For this review, take the finished solid that the model builds, in its own axes (mm). A direction names the side the tool comes from. Coordinates: 2 decimals unless noted, no trailing zeros. Write each loop counter-clockwise with the first axis right and the second up, starting at its lowest first coordinate (ties: lowest second). Pieces come first, ordered by that corner, then holes. Notation, with made-up numbers: (38, 84.5) -> (45, 84.5) arc R20 ccw to (45, 89.5) -> close; hole circle Ø5 at (-32, -8.75). An arc over 180 degrees is marked (long way). Put each result on its own line as item: value. Start each with the question number.
Item 1: For faces 5 (the flat face through (12, -3, 1)), 6 (the cylindrical face through (17.456, 0.011, 3.857)), list the 3-axis set-ups (+Z, -Z, +X, -X, +Y, -Y) from which the entire face can be reached by the end or side of a thin tool; tool diameter is ignored.
Item 2: Consider section A-A on x = 16.25. Give the boundary of the cut face in (y, z).
Item 3: Insertion check: P1, Ø1.8, axis at x = 15, z = 4, coming from the +Y side; P2, Ø2.5, axis at x = 15.5, z = 3.5, coming from the -Y side. Each pin has a flat end and moves straight along its axis. Give the tip position at first contact, or say it passes through.
Item 4: Consider section C-C on y = -0.25. Give the boundary of the cut face in (x, z).
Item 5: Consider section B-B on z = 1.6. Give the boundary of the cut face in (x, y), and give its area (3 significant figures).
Item 6: The part is to be moulded in two halves that separate along X. For faces 1 (the flat face through (15, 0.5, 4)), 2 (the flat face through (18.456, 0, 3)), 3 (the flat face through (12, 0, 0)), 4 (the flat face through (15, -0.5, 4)), say which applies: +X half, -X half, draft (parallel to the pull), parting line (faces both ways), or undercut.
Item 7: To check wall thickness, follow L1, parallel to Y at x = 15.75, z = 0.4; L2, parallel to X at y = 0.25, z = 4.15; L3, parallel to Y at x = 18, z = 2.45. State the ranges of each line that lie inside material, in increasing order.
```python
from build123d import *

# Parameters (mm, degrees)
F0_W     = 12
F0_H     = 6
F1_DEPTH = 5
F2_R     = 2.99999
F3_R     = 1.25
F4_DEPTH = 25
F6_DEPTH = 25


# Not quite as in the source:
# - a fillet or chamfer is up to 0.001 mm smaller than in the source, because OpenCascade refuses the exact size


with BuildPart() as f1:
    # F0 (on Top) → F1 (new body)
    with BuildSketch(Plane.XY):
        with Locations((12.4557307512, 0)):
            Rectangle(F0_W, F0_H)
    extrude(amount=F1_DEPTH)

    # F2 (radius 3 in the source; OpenCascade refuses exactly that, so slightly less here)
    f2_edges = [f1.edges().sort_by_distance(p)[0] for p in [
        (12.455731, -3, 5),
        (12.455731, 3, 5),
    ]]
    fillet(f2_edges, radius=F2_R)

    # F3 (on face) → F4 (cut)
    with BuildSketch(Plane.YZ.offset(18.4557307512)):
        with Locations((0, 1.6)):
            Circle(F3_R)
    extrude(amount=-F4_DEPTH, mode=Mode.SUBTRACT)

    # F5 (on face) → F6 (cut)
    with BuildSketch(Plane(origin=(0, 0, 0), x_dir=(1, 0, 0), z_dir=(0, 0, -1))):
        with BuildLine():
            Line((13.9557307512, -0.5), (16.9557307512, -0.5))
            ThreePointArc((16.9557307512, -0.5), (17.4557307512, 0), (16.9557307512, 0.5))
            Line((16.9557307512, 0.5), (13.9557307512, 0.5))
            ThreePointArc((13.9557307512, 0.5), (13.4557307512, 0), (13.9557307512, -0.5))
        make_face()
    extrude(amount=-F6_DEPTH, mode=Mode.SUBTRACT)


solid = f1.part
```
Return value:
1. face 5: +Z, -Z, +X, -X, -Y
1. face 6: +Z, -Z
2. outline: (-3, 0) -> (-0.5, 0) -> (-0.5, 0.45) arc R1.25 cw to (-0.5, 2.75) -> (-0.5, 4.96) arc R3 ccw to (-3, 2) -> close; (0.5, 0) -> (3, 0) -> (3, 2) arc R3 ccw to (0.5, 4.96) -> (0.5, 2.75) arc R1.25 cw to (0.5, 0.45) -> close
3. P1: y = 2.79
3. P2: y = -2.99
4. outline: (6.46, 0) -> (13.52, 0) -> (13.52, 0.38) -> (6.46, 0.38) -> close; (6.46, 2.82) -> (13.52, 2.82) -> (13.52, 4.99) -> (6.46, 4.99) -> close; (17.39, 0) -> (18.46, 0) -> (18.46, 0.38) -> (17.39, 0.38) -> close; (17.39, 2.82) -> (18.46, 2.82) -> (18.46, 4.99) -> (17.39, 4.99) -> close
5. outline: (6.46, -3) -> (18.46, -3) -> (18.46, -1.25) -> (6.46, -1.25) -> close; (6.46, 1.25) -> (18.46, 1.25) -> (18.46, 3) -> (6.46, 3) -> close
5. area: 42.0 mm^2
6. face 1: undercut
6. face 2: +X half
6. face 3: draft
6. face 4: undercut
7. L1: -3 to -0.5, 0.5 to 3
7. L2: 6.46 to 13.52, 17.39 to 18.46
7. L3: -2.97 to -0.92, 0.92 to 2.97
